Source: three-view drawing plus pictorial views. Frame: mm from the lowest corner of the part. Give positions to 0.01 mm unless a question says otherwise; leave off trailing zeros. Order: outer loops, then holes, each group sorted by start corner. A loop starts at its lowest first (then second) coordinate and runs counter-clockwise, first axis right, second up. Notation, with made-up numbers: (-10.75, 69) -> (20.25, 69) arc R17 ccw to (20.25, 75) -> close; hole circle Ø1 at (-9.5, -5.5). An arc over 180 degrees is marked (long way). Answer in a Markdown table with one row per item. Add a question column.
Q1. Cut plane A-A on x = 1.5. Return the cut outline in (y, z).
Q2. Line query: line 1 along Z through (x, y) = (3.7, 29); line 2 along Y through (x, z) = (0.6, 29); line 3 along Z through (x, y) = (1.7, 29). Output: solid intervals per line, ascending. Write a range as from..to.
Q3. Contact query for flat-ended pins moving along their axis: P1, Ø3, axis at x = 8, z = 8.5, coming from the -Y side; P2, Ø4, axis at x = 10.5, z = 52, coming from the -Y side; P3, Ø12, axis at x = 14, z = 46, coming from the +Y side. Output: stop coordinate, or through.
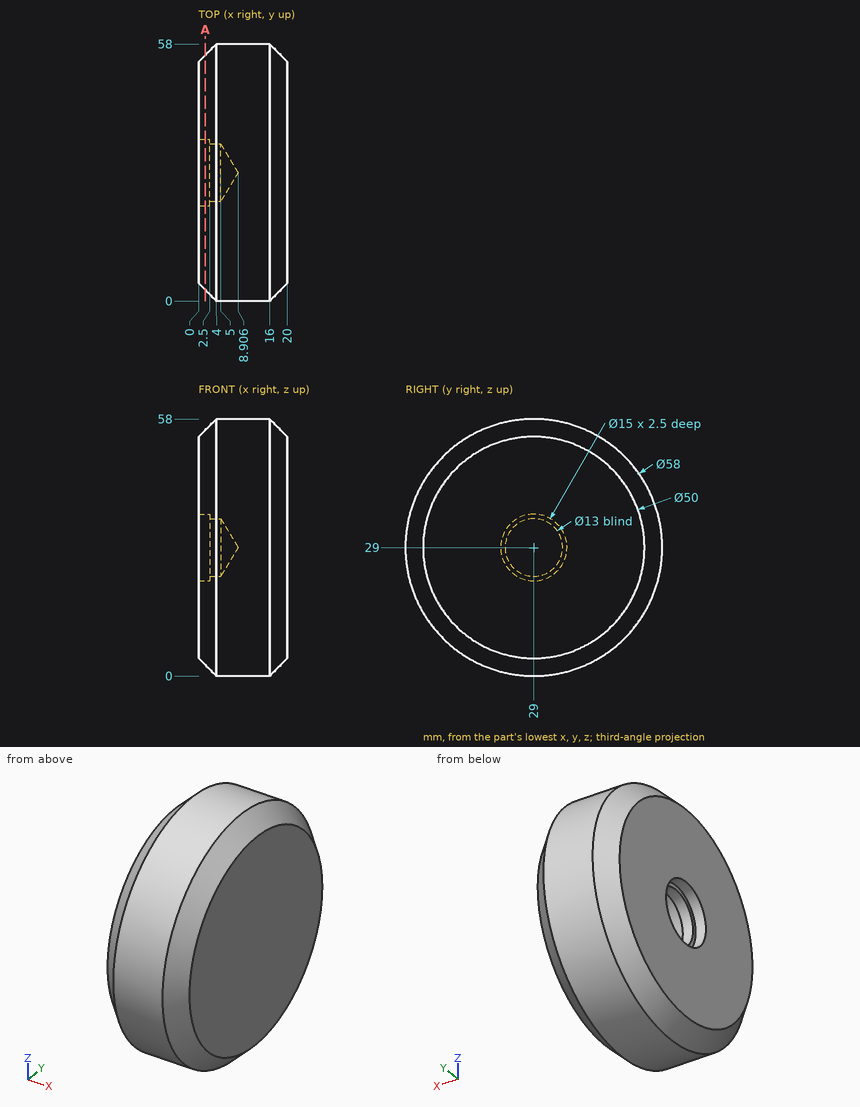
Completed:
| question | item | result |
|---|---|---|
| 1 | outline | circle Ø53 at (29, 29); hole circle Ø15 at (29, 29) |
| 2 | line 1 | z = 0.3..22.5, 35.5..57.7 |
| 2 | line 2 | y = 3.4..21.5, 36.5..54.6 |
| 2 | line 3 | z = 2.3..21.5, 36.5..55.7 |
| 3 | P1 | stops at y = 7.09 |
| 3 | P2 | stops at y = 9 |
| 3 | P3 | stops at y = 55.83 |
